```python
from build123d import *

# Parameters (mm, degrees)
SKETCH1_R           = 30
SKETCH1_R_2         = 21.5
BOSS_EXTRUDE1_DEPTH = 14
SKETCH2_R           = 30
SKETCH2_R_2         = 2.125
SKETCH2_R_3         = 13.25
BOSS_EXTRUDE2_DEPTH = 3
SKETCH4_R           = 1.625
CUT_EXTRUDE1_DEPTH  = 46.705579528


with BuildPart() as part:
    # Sketch1 → Boss-Extrude1 (new body)
    with BuildSketch(Plane(origin=(0, 0, 0), x_dir=(0, 0, -1), z_dir=(1, 0, 0))):
        Circle(SKETCH1_R)
        Circle(SKETCH1_R_2, mode=Mode.SUBTRACT)
    extrude(amount=BOSS_EXTRUDE1_DEPTH)

    # Sketch2 → Boss-Extrude2 (add)
    with BuildSketch(Plane(origin=(14, 0, 0), x_dir=(0, 0, -1), z_dir=(1, 0, 0))):
        Circle(SKETCH2_R)
        with Locations((0, 17.5)):
            Circle(SKETCH2_R_2, mode=Mode.SUBTRACT)
        with Locations((17.5, 0)):
            Circle(SKETCH2_R_2, mode=Mode.SUBTRACT)
        with Locations((0, -17.5)):
            Circle(SKETCH2_R_2, mode=Mode.SUBTRACT)
        with Locations((-17.5, 0)):
            Circle(SKETCH2_R_2, mode=Mode.SUBTRACT)
        Circle(SKETCH2_R_3, mode=Mode.SUBTRACT)
    extrude(amount=BOSS_EXTRUDE2_DEPTH)

    # Sketch4 → Cut-Extrude1 (cut, through all)
    with BuildSketch(Plane(origin=(17, 0, 0), x_dir=(0, 0, -1), z_dir=(1, 0, 0))):
        with Locations((-20.175789947, 16)):
            Circle(SKETCH4_R)
        with Locations((16, 20.175789947)):
            Circle(SKETCH4_R)
        with Locations((20.175789947, -16)):
            Circle(SKETCH4_R)
        with Locations((-16, -20.175789947)):
            Circle(SKETCH4_R)
    extrude(amount=-CUT_EXTRUDE1_DEPTH, mode=Mode.SUBTRACT)


solid = part.part
```
For this review, take the finished solid that the model builds, in its own axes (mm). A direction names the side the tool comes from. Coordinates: 2 decimals unless noted, no trailing zeros. Order: outer loops, then holes, each group sorted by start corner. A loop starts at its lowest first (then second) coordinate and runs counter-clockwise, first axis right, second up. Notation, with made-up numbers: (-4, 47.5) - (50, 47.5) arc R7 cw to (50, 55.5) - close; hole circle Ø6 at (4.25, -13.75). An arc over 180 degrees is marked (long way). Answer as a JSON object with one key per item and string values. Group by question number.
1. For probe 1 along Y at (x, z) = (15.6, 0) (3 decimals); probe 2 along Z at (x, y) = (12.25, -19); probe 3 along Y at (x, z) = (9.25, 15.5), list the stretches that pass through material, from the lowest coordinate up.
2. We need section A-A on y = 0. State the section outline as (x, z) points (3 decimals), then the cut area to 3 significant figures.
3. We need section D-D on x = 15.25. Give the number of separate pieces and of enclosed holes in the cut face, then the cut area to 3 significant figures.
4. For faces 4 (the cylindrical face through (8.619, 14.558, 19.426)), 5 (the flat face through (14, 10, -9)), list the 3-axis set-ups (+Z, -Z, +X, -X, +Y, -Y) from which the entire face can be reached by the end or side of a thin tool; tool diameter is ignored.
5. Clearance check with flat-ended pins moving along their axes: P1, Ø1.5, axis at x = 14, z = -12, coming from the -Y side; P2, Ø2, axis at x = 8, z = 21, coming from the +Y side; P3, Ø10, axis at x = 14, y = 22.5, coming from the +Z side; P4, Ø21, axis at y = 0, z = 0, coming from the -X side. State where each tip first meets the part, or that it passes through.
6. The part is to be moulded in two halves that separate along Y. For faces 1 (the cylindrical face through (6.902, 21.317, 2.799)), 2 (the cylindrical face through (8.38, 1.32, 29.97)), 3 (the flat face through (0, -20, -13)), say which applies: pulls with the +Y half, pulls with the -Y half, needs draft (parallel to the pull), parting line crosses it, or undercut.
7. We need section B-B on z = 3. State the section outline as (x, y) points, then the cut area to 3 significant figures.
8. We need section C-C on y = 6. State the section outline as (x, z) points.
Final values:
{
 "1": {"probe 1": "-30 to -19.625, -15.375 to -13.25, 13.25 to 15.375, 19.625 to 30", "probe 2": "-23.22 to -10.06, 10.06 to 14.88, 17.12 to 23.22", "probe 3": "-25.69 to -21.72, -18.63 to -14.9, 14.9 to 25.69"},
 "2": {"outline": "(0, -30) - (17, -30) - (17, -19.625) - (14, -19.625) - (14, -21.5) - (0, -21.5) - close; (0, 21.5) - (14, 21.5) - (14, 19.625) - (17, 19.625) - (17, 30) - (0, 30) - close; (14, -15.375) - (17, -15.375) - (17, -13.25) - (14, -13.25) - close; (14, 13.25) - (17, 13.25) - (17, 15.375) - (14, 15.375) - close", "area": "313 mm²"},
 "3": {"separate pieces": "1", "enclosed holes": "9", "area": "2,190 mm²"},
 "4": {"face 4": "+X, -X", "face 5": "-X"},
 "5": {"P1": "y = -27.81", "P2": "y = 22.36", "P3": "z = 24.37", "P4": "through"},
 "6": {"face 1": "undercut", "face 2": "parting line crosses it", "face 3": "needs draft"},
 "7": {"outline": "(0, -29.85) - (17, -29.85) - (17, -12.91) - (14, -12.91) - (14, -21.29) - (0, -21.29) - close; (0, 21.29) - (14, 21.29) - (14, 12.91) - (17, 12.91) - (17, 29.85) - (0, 29.85) - close", "area": "341 mm²"},
 "8": {"outline": "(0, -29.39) - (17, -29.39) - (17, -11.81) - (14, -11.81) - (14, -20.65) - (0, -20.65) - close; (0, 20.65) - (14, 20.65) - (14, 11.81) - (17, 11.81) - (17, 29.39) - (0, 29.39) - close"}
}
